Can you work these out from the model? Positions are in its coordinate system, mm. Coordinates: 2 decimals unless noted, no trailing zeros. Loops run counter-clockwise (first coordinate to the right, second up) from the corner with the lowest first, then second, coordinate; pieces in that order, holes last.
```python
from build123d import *

# Parameters (mm, degrees)
SKETCH1_R           = 1.7
SKETCH1_R_2         = 1.125
BOSS_EXTRUDE1_DEPTH = 4


with BuildPart() as part:
    # Sketch1 → Boss-Extrude1 (new body)
    with BuildSketch(Plane(origin=(0, 0, 0), x_dir=(1, 0, 0), z_dir=(0, 1, 0))):
        with BuildLine():
            Line((-1.861032186, 5.671500837), (11.70980962, 13.943858026))
            ThreePointArc((11.70980962, 13.943858026), (11.793110745, 14.390229161), (11.926465203, 14.824283138))
            ThreePointArc((11.926465203, 14.824283138), (12.627588108, 16.022788534), (13.696191423, 16.909397504))
            Line((13.696191423, 16.909397504), (31.922238344, 27.299860881))
            ThreePointArc((31.922238344, 27.299860881), (37.378259624, 25.805929226), (35.88432797, 20.349907946))
            Line((35.88432797, 20.349907946), (17.658281049, 9.95944457))
            ThreePointArc((17.658281049, 9.95944457), (16.016619967, 9.448844707), (14.312262761, 9.674521117))
            Line((14.312262761, 9.674521117), (0.741420954, 1.402163927))
            ThreePointArc((0.741420954, 1.402163927), (-2.694474071, 2.235605811), (-1.861032186, 5.671500837))
        make_face()
        with Locations(Location((15.677236236, 13.434421037, 0), (0, 0, 270))):
            Circle(SKETCH1_R, mode=Mode.SUBTRACT)
        with Locations(Location((33.903283157, 23.824884413, 0), (0, 0, 270))):
            Circle(SKETCH1_R, mode=Mode.SUBTRACT)
        with Locations(Location((-0.559805616, 3.536832382, 0), (0, 0, 270))):
            Circle(SKETCH1_R_2, mode=Mode.SUBTRACT)
    extrude(amount=BOSS_EXTRUDE1_DEPTH)


solid = part.part
```
Item 1: Suppose I cut it at D-D, the plane x = 27. Please give me the cut outline in (y, z).
Results are:
outline: (0, -24.49) - (4, -24.49) - (4, -15.29) - (0, -15.29) - close
Item 2: Suppose I cut it at B-B, the plane y = 2.8. Count the separate pieces of the cut face and the enclosed holes in it, plus the area to 3 significant figures.
Results are:
separate pieces: 1
enclosed holes: 3
area: 282 mm2
Item 3: Suppose I cut it at A-A, the plane z = -12.75. Please give me the cut outline in (x, y).
Results are:
outline: (9.75, 0) - (14.12, 0) - (14.12, 4) - (9.75, 4) - close; (17.23, 0) - (22.55, 0) - (22.55, 4) - (17.23, 4) - close
Item 4: Suppose I cut it at C-C, the plane z = -22.75. Please give me the cut outline in (x, y).
Results are:
outline: (23.94, 0) - (32.59, 0) - (32.59, 4) - (23.94, 4) - close; (35.22, 0) - (37.76, 0) - (37.76, 4) - (35.22, 4) - close
Item 5: We'd pull the mould along Z, two halves only. Please class faces 1 (the face through (33.978, 1.972, -25.523)), 2 (the face through (26.9, 1.97, -15.23)), 3 (the face through (19, 4, -15)), 4 (the face through (-1.244, 1.972, -4.43)): +Z half, -Z half, draft (parallel to the pull), parting line (faces both ways), or undercut.
Results are:
face 1: undercut
face 2: +Z half
face 3: draft
face 4: undercut
Item 6: I'm going to push flat-ended pins straight in: P1, Ø1.3, axis at x = -0.56, z = -3.54, coming from the +Y side; P2, Ø1, axis at y = 2.5, z = -8.5, coming from the -X side. Where does each tip first touch, or does it pass through?
Results are:
P1: passes through
P2: stops at x = 1.96
Item 7: I need wall thicknesses on line 1 along X through (y, z) = (3.6, -3.75); line 2 along X through (y, z) = (3.3, -22.5); line 3 along X through (y, z) = (2, -9). Which ranges of each line are inside material? Lowest first, please.
Results are:
line 1: x = -3.05 to -1.66, 0.54 to 4.59
line 2: x = 23.5 to 32.84, 34.97 to 37.68
line 3: x = 3.6 to 13.21
